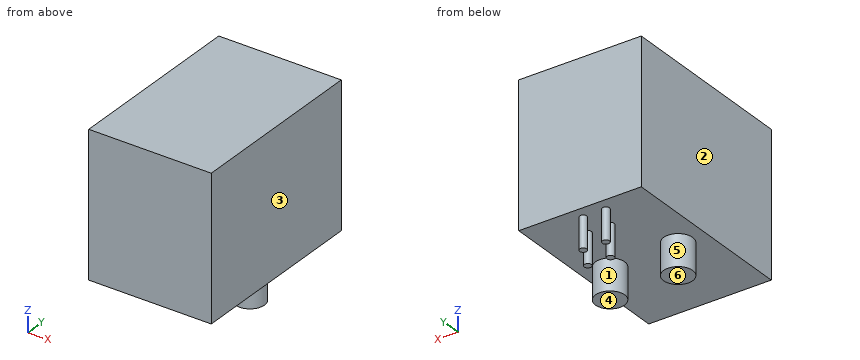
```python
from build123d import *

# Parameters (mm, degrees)
F0_W     = 13.72
F0_H     = 20.6
F1_DEPTH = 16
F2_R     = 1.625
F3_DEPTH = 3.5
F4_R     = 0.4
F5_DEPTH = 3.5


with BuildPart() as f1:
    # F0 (on Top) → F1 (new body)
    with BuildSketch(Plane.XY):
        Rectangle(F0_W, F0_H)
    extrude(amount=F1_DEPTH)

    # F2 (on face) → F3 (join)
    with BuildSketch(Plane(origin=(0, 0, 0), x_dir=(1, 0, 0), z_dir=(0, 0, -1))):
        with Locations((-3.81, -0.14)):
            Circle(F2_R)
        with Locations((3.81, -0.14)):
            Circle(F2_R)
    extrude(amount=F3_DEPTH)

    # F4 (on face) → F5 (join)
    with BuildSketch(Plane(origin=(0, 0, 0), x_dir=(1, 0, 0), z_dir=(0, 0, -1))):
        with Locations((-0.635, -6.35)):
            Circle(F4_R)
        with Locations((1.905, -6.35)):
            Circle(F4_R)
        with Locations((-1.905, -8.89)):
            Circle(F4_R)
        with Locations((0.635, -8.89)):
            Circle(F4_R)
    extrude(amount=F5_DEPTH)


solid = f1.part
```
Can you work these out from the model? Positions are in its coordinate system, mm. Face numbers are marked on the shaded views. A direction names the side the tool comes from. Give positions to 0.01 mm unless a question says otherwise; leave off trailing zeros. Loops run counter-clockwise (first coordinate to the right, second up) from the corner with the lowest first, then second, coordinate; pieces in that order, holes last. Notation, with made-up numbers: M -9,-0.5 L 7,-0.5 A28 ccw 7,38.5 Z; hole C 65.25,53 d2. An arc over 180 degrees is marked long. Use one line per item in the form item = value. Start each with the question number.
(1) I want a section at A-A, the plane y = 0.14. Write out the boundary of the cut face in (x, z) (3 decimals).
(2) I'm going to push a flat-ended pin straight in: P1, Ø4, axis at x = -3.5, y = -7.5, coming from the -Z side. Where does the tip first touch, or does it pass through?
(3) I want a section at C-C, the plane x = 5.75. Write out the boundary of the cut face in (y, z), and give its area (3 significant figures).
(4) I want a section at B-B, the plane z = -0.5. Write out the boundary of the cut face in (x, y) (3 decimals).
(5) Please list where these lines run through material, in increasing order: line 1 (Z direction, x = -0.75, y = 0.75); line 2 (X direction, y = 0.5, z = -2.25).
(6) I want a section at D-D, the plane y = 8.89. Write out the boundary of the cut face in (x, z) (3 decimals).
(7) Thinking about a two-plate mould opening in X: for the marked faces 1, 2, 3 and 4, which applies, released by +X, released by -X, zero draft, split by the parting line, or undercut?
(8) On a 3-axis mill with a long thin cutter (end or side, diameter ignored), from which of +Z, -Z, +X, -X, +Y, -Y can I reach the whole of each face in a straight line? I mean the marked faces 5 and 6. Say none if no direction works.
Worked out:
q1.outline = M -6.86,0 L -5.435,0 L -5.435,-3.5 L -2.185,-3.5 L -2.185,0 L 2.185,0 L 2.185,-3.5 L 5.435,-3.5 L 5.435,0 L 6.86,0 L 6.86,16 L -6.86,16 Z
q2.P1 = 0
q3.outline = M -10.3,0 L 10.3,0 L 10.3,16 L -10.3,16 Z
q3.area = 330 mm²
q4.outline = C -3.81,0.14 d3.25; C -1.905,8.89 d0.8; C -0.635,6.35 d0.8; C 0.635,8.89 d0.8; C 1.905,6.35 d0.8; C 3.81,0.14 d3.25
q5.line_1 = 0 to 16
q5.line_2 = -5.39 to -2.23, 2.23 to 5.39
q6.outline = M -6.86,0 L -2.305,0 L -2.305,-3.5 L -1.505,-3.5 L -1.505,0 L 0.235,0 L 0.235,-3.5 L 1.035,-3.5 L 1.035,0 L 6.86,0 L 6.86,16 L -6.86,16 Z
q7.face_1 = undercut
q7.face_2 = released by -X
q7.face_3 = released by +X
q7.face_4 = zero draft
q8.face_5 = -Z
q8.face_6 = -Z, +X, -X, +Y, -Y
